Source: CAD feature listing. Evaluate the final solid. Frame: model axes, mm. A direction names the side the tool comes from. Coordinates: 2 decimals unless noted, no trailing zeros. Write each loop counter-clockwise with the first axis right and the second up, starting at its lowest first coordinate (ties: lowest second). Pieces come first, ordered by that corner, then holes. Notation, with made-up numbers: (-3, 84) -> (11, 84) arc R15 cw to (11, 95) -> close; hole circle Ø2 at (-9.75, 9.25). An arc over 180 degrees is marked (long way). One line per item, written item: value. Start each with the question number.
1. Section query C-C, the plane y = 7.75. Output: boundary loops of the cut face in (x, z), and give its area (3 significant figures).
2. First-contact query: P1, Ø8, axis at x = -1.5, z = 0, coming from the -Y side; P2, Ø2.5, axis at y = 7.5, z = -2.5, coming from the +X side; P3, Ø6, axis at x = -16, y = 0, coming from the +Z side. Flat tips, straight axial feed; report the tip coordinate or a pass-through.
3. Section query B-B, the plane x = 11. Output: boundary loops of the cut face in (y, z).
4. Access query for faces 4 (the flat face through (0, 0, 0)), 5 (the flat face through (20, -4, -6)), 6 (the cylindrical face through (-5.437, 1.395, 17.264)), 7 (the flat face through (-20, -4, -6)). Directions: +Z, -Z, +X, -X, +Y, -Y. A direction counts if a zero-diameter tool reaches every point of the face in a straight line with its end or side. Return the directions, or none.
5. Line query: line 1 (X direction, y = -3.9, z = 0); line 2 (Y direction, x = -2, z = 10); line 3 (X direction, y = -5, z = -11). Output: solid intervals per line, ascending.
6. Section query A-A, the plane z = 0. Output: boundary loops of the cut face in (x, y).
7. Section query D-D, the plane y = 5. Output: boundary loops of the cut face in (x, z).
8. Mould query, pull axis Z, two halves, no side actions, for faces 1 (the flat face through (-23, -4, 0)), 2 (the flat face through (-20, -4, 6)), 3 (the flat face through (0, 6, 0)). Classes: released by +Z, released by -Z, zero draft, split by the parting line, or undercut.
from build123d import *

# Parameters (mm, degrees)
CROQUIS2_W              = 21
CROQUIS2_H              = 16
CORTAR_EXTRUIR1_DEPTH   = 3
CROQUIS4_W              = 8
CROQUIS4_H              = 12
CROQUIS4_R              = 1.5
SALIENTE_EXTRUIR1_DEPTH = 5


with BuildPart() as part:
    # Croquis1 → Revolución1 (revolve)
    with BuildSketch(Plane.XY, mode=Mode.PRIVATE) as revoluci_n1_sk:
        Polygon((-18.1, 9), (-18.1, -6), (-13.1, -6), (-13.1, 0), (0, 0), (0, 9), align=None)
    revolve(revoluci_n1_sk.sketch.rotate(Axis((0, 25.323006639, 0), (0, -1, 0)), 270), axis=Axis((0, 25.323006639, 0), (0, -1, 0)))

    # Croquis2 → Cortar-Extruir1 (cut)
    with BuildSketch(Plane(origin=(0, 9, 0), x_dir=(1, 0, 0), z_dir=(0, 1, 0))):
        Rectangle(CROQUIS2_W, CROQUIS2_H)
    extrude(amount=-CORTAR_EXTRUIR1_DEPTH, mode=Mode.SUBTRACT)

    # Croquis4 → Saliente-Extruir1 (add)
    # profile 1 of 2: a face of its own
    with BuildSketch(Plane.XZ.offset(6)):
        with Locations((-19, 0)):
            Rectangle(CROQUIS4_W, CROQUIS4_H)
        with Locations(Location((-20.333333333, 0, 0), (0, 0, 270))):
            Circle(CROQUIS4_R, mode=Mode.SUBTRACT)
    # profile 2 of 2: a face of its own
    with BuildSketch(Plane.XZ.offset(6)):
        with Locations((19, 0)):
            Rectangle(CROQUIS4_W, CROQUIS4_H)
        with Locations(Location((20.333333333, 0, 0), (0, 0, 90))):
            Circle(CROQUIS4_R, mode=Mode.SUBTRACT)
    extrude(amount=-SALIENTE_EXTRUIR1_DEPTH)


solid = part.part
Computed values:
1. outline: circle Ø36.2 at (0, 0); hole (-10.5, -8) -> (10.5, -8) -> (10.5, 8) -> (-10.5, 8) -> close
1. area: 693 mm²
2. P1: stops at y = 0
2. P2: stops at x = 18.06
2. P3: stops at z = 12.59
3. outline: (-6, -14.37) -> (9, -14.37) -> (9, 14.37) -> (-6, 14.37) -> (-6, 7.11) -> (0, 7.11) -> (0, -7.11) -> (-6, -7.11) -> close
4. face 4: -Y
4. face 5: -Z, +X, +Y, -Y
4. face 6: +Y
4. face 7: -Z, -X, +Y, -Y
5. line 1: x = -23 to -21.83, -18.83 to -13.1, 13.1 to 18.83, 21.83 to 23
5. line 2: y = 0 to 9
5. line 3: x = -14.37 to -7.11, 7.11 to 14.37
6. outline: (-23, -6) -> (-21.83, -6) -> (-21.83, -1) -> (-23, -1) -> close; (-18.83, -6) -> (-13.1, -6) -> (-13.1, 0) -> (13.1, 0) -> (13.1, -6) -> (18.83, -6) -> (18.83, -1) -> (18.1, -1) -> (18.1, 9) -> (10.5, 9) -> (10.5, 6) -> (-10.5, 6) -> (-10.5, 9) -> (-18.1, 9) -> (-18.1, -1) -> (-18.83, -1) -> close; (21.83, -6) -> (23, -6) -> (23, -1) -> (21.83, -1) -> close
7. outline: circle Ø36.2 at (0, 0)
8. face 1: zero draft
8. face 2: released by +Z
8. face 3: undercut
